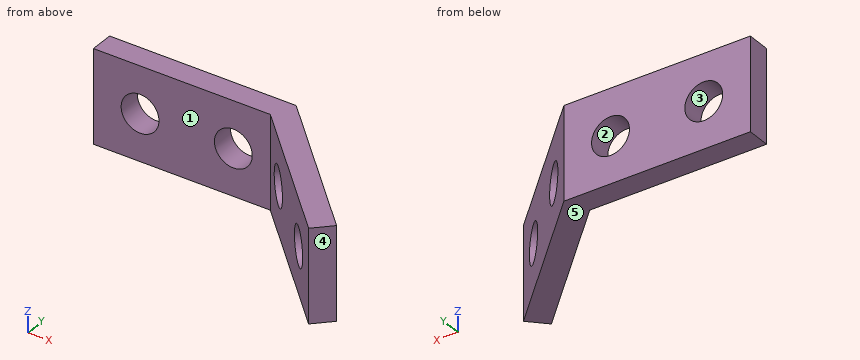
from build123d import *

# Parameters (mm, degrees)
BOSS_EXTRUDE1_DEPTH = 12.7
SKETCH2_R           = 2.5796875
CUT_EXTRUDE1_DEPTH  = 12.7
SKETCH3_R           = 2.5796875
CUT_EXTRUDE2_DEPTH  = 12.7


with BuildPart() as part:
    # Sketch1 → Boss-Extrude1 (new body)
    with BuildSketch(Plane.XY):
        Polygon((-102.370082778, 43.999509732), (-76.970082778, 43.999509732), (-59.009570536, 26.03899749), (-61.254634567, 23.79393346), (-78.285210839, 40.824509732), (-102.370082778, 40.824509732), align=None)
    extrude(amount=BOSS_EXTRUDE1_DEPTH)

    # Sketch2 → Cut-Extrude1 (cut)
    with BuildSketch(Plane(origin=(0, 43.999509732, 0), x_dir=(1, 0, 0), z_dir=(0, 1, 0))):
        with Locations(Location((-96.020082778, -6.35, 0), (0, 0, 180))):
            Circle(SKETCH2_R)
        with Locations(Location((-83.320082778, -6.35, 0), (0, 0, 180))):
            Circle(SKETCH2_R)
    extrude(amount=-CUT_EXTRUDE1_DEPTH, mode=Mode.SUBTRACT)

    # Sketch3 → Cut-Extrude2 (cut)
    with BuildSketch(Plane(origin=(-16.485286523, -16.485286523, 0), x_dir=(0, 0, -1), z_dir=(0.707106781186552, 0.707106781186543, 0))):
        with Locations(Location((-6.35, 66.488419182, 0), (0, 0, 90))):
            Circle(SKETCH3_R)
        with Locations(Location((-6.35, 79.188419182, 0), (0, 0, 90))):
            Circle(SKETCH3_R)
    extrude(amount=-CUT_EXTRUDE2_DEPTH, mode=Mode.SUBTRACT)


solid = part.part
Verification items for the finished model (mm, model axes). Face numbers are marked on the shaded views. A direction names the side the tool comes from. Give positions to 0.01 mm unless a question says otherwise; leave off trailing zeros. Order: outer loops, then holes, each group sorted by start corner. A loop starts at its lowest first (then second) coordinate and runs counter-clockwise, first axis right, second up. Notation, with made-up numbers: M 59,46 L 106,46 A16 ccw 106,50 Z; hole C 5.5,-28.5 d10. An arc over 180 degrees is marked long. Use one line per item in the form item = value. Start each with the question number.
Q1. Section check A-A (z = 6.35). Enter the section's corners in (x, y).
Q2. Section check C-C (x = -80). Enter the section's corners in (y, z), then the cut area to 3 significant figures.
Q3. Scan lines: line 1 along Y through (x, z) = (-93, 11.75); line 2 along X through (y, z) = (26.75, 7.5); line 3 along Y through (x, z) = (-72.5, 12.25). Record each from-to range of solid material in increasing order. Write a range as [from, to].
Q4. Mould release check, pull along X, two halves, no side actions. Record for the marked faces 3, 4 and 5: +X half, -X half, draft (parallel to the pull), parting line (faces both ways), or undercut.
Q5. Section check D-D (y = 33.5). Enter the section's corners in (x, z).
Q6. Access from +Z, -Z, +X, -X, +Y, -Y to the whole of each face (thin tool, end or side, straight path). Record for the marked faces 1 and 2.
Q7. Go/stop test with flat-tipped pins: pin 1 Ø2 at (x, z) = (-73, 1.5) entering from +Y; pin 2 Ø3 at (x, z) = (-71, 9) entering from -Y; pin 3 Ø4 at (y, z) = (37.5, 8) entering from +X; pin 4 Ø4.5 at (x, z) = (-83.32, 6.35) entering from -Y. Record where each tip stops, or that it passes through.
Q8. Section check B-B (x = -85). Enter the section's corners in (y, z).
Evaluation:
q1.outline = M -102.37,40.82 L -98.6,40.82 L -98.6,44 L -102.37,44 Z; M -93.44,40.82 L -85.9,40.82 L -85.9,44 L -93.44,44 Z; M -80.74,40.82 L -78.29,40.82 L -76.55,39.09 L -74.3,41.33 L -76.97,44 L -80.74,44 Z; M -72.9,35.44 L -67.57,30.11 L -65.32,32.35 L -70.66,37.69 Z; M -63.92,26.46 L -61.25,23.79 L -59.01,26.04 L -61.68,28.71 Z
q2.outline = M 40.82,0 L 44,0 L 44,12.7 L 40.82,12.7 Z
q2.area = 40.3 mm2
q3.line_1 = [40.82, 44]
q3.line_2 = [-64.01, -59.72]
q3.line_3 = [35.04, 39.53]
q4.face_3 = undercut
q4.face_4 = +X half
q4.face_5 = draft
q5.outline = M -70.96,0 L -66.47,0 L -66.47,12.7 L -70.96,12.7 Z
q6.face_1 = +Z, -Z, -X, -Y
q6.face_2 = +Y, -Y
q7.pin_1 = 41.03
q7.pin_2 = 32.04
q7.pin_3 = -68.47
q7.pin_4 = through
q8.outline = M 40.82,0 L 44,0 L 44,4.39 L 40.82,4.39 Z; M 40.82,8.31 L 44,8.31 L 44,12.7 L 40.82,12.7 Z
